For this review, take the finished solid that the model builds, in its own axes (mm). Coordinates: 2 decimals unless noted, no trailing zeros. Loops run counter-clockwise (first coordinate to the right, second up) from the corner with the lowest first, then second, coordinate; pieces in that order, holes last. Notation, with made-up numbers: (76.5, 5) - (105.5, 5) arc R32 ccw to (105.5, 33) - close; hole circle Ø2 at (56, -26.75). An arc over 180 degrees is marked (long way). One line per item, written item: value. Start each with the question number.
1. To check wall thickness, follow line 1 (Y direction, x = 0, z = 8.75) (3 decimals); line 2 (Y direction, x = 0, z = 10.25) (3 decimals); line 3 (Z direction, x = -1.5, y = -0.5). State the ranges of each line that lie inside material, in increasing order. Write a range as from..to.
2. Insertion check: pin 1 (7 mm diameter, centred on x = 0, y = 0, fed in from +Z); pin 2 (6 mm diameter, centred on x = 1, y = -2.5, fed in from +Z); pin 3 (3 mm diameter, centred on y = -4.5, z = 5.5, fed in from +X); pin 4 (6 mm diameter, centred on y = -2, z = 0, fed in from +X). Each pin has a flat end and moves straight along its axis. Give the tip position at first contact, or say it passes through.
3. Take a section at D-D, the plane z = -0.5. State the section outline as (x, y) points, and give its area (3 significant figures).
4. Take a section at C-C, the plane z = 4.75. State the section outline as (x, y) points (3 decimals).
5. Take a section at A-A, the plane y = 0. State the section outline as (x, z) points (3 decimals).
6. The part is to be moulded in two halves that separate along Y. For faces 1 (the face through (0, 0, 4)), 2 (the face through (4, -4, 9)), 3 (the face through (6.466, 2.681, 10.479)), 4 (the face through (4.125, 1.299, 8.056)), say which applies: released by +Y, released by -Y, zero draft, split by the parting line, or undercut.
Autodesk Inventor part; units mm, degrees
ref_plane "YZ Plane" through (0, 0, 0) normal (1, 0, 0) x (0, 1, 0)
ref_plane "XZ Plane" through (0, 0, 0) normal (0, 1, 0) x (-1, 0, 0)
ref_plane "XY Plane" through (0, 0, 0) normal (0, 0, 1) x (1, 0, 0)
sketch "Sketch5" plane through (0, 0, 0) normal (0, 0, 1) x (1, 0, 0)
  circle A0 centre (0, 0) radius 5.45
  dimension "d0" = 10.9
extrude "Extrusion1" add sketch "Sketch5" along normal blind 9
sketch "Sketch6" plane through (0, 0, 9) normal (0, 0, 1) x (1, 0, 0)
  circle A0 centre (0, 0) radius 7
  dimension "d3" = 14
extrude "Extrusion2" add sketch "Sketch6" along normal blind 3
sketch "Sketch7" plane through (0, 0, 12) normal (0, 0, 1) x (1, 0, 0)
  circle A0 centre (0, 0) radius 4.325
  dimension "d6" = 8.65
extrude "Extrusion3" cut sketch "Sketch7" against normal blind 8
sketch "Sketch8" plane through (0, 0, 0) normal (0, 0, -1) x (-1, 0, 0)
  circle A0 centre (0, 0) radius 5.45
  dimension "d9" = 10.9
extrude "Extrusion4" add sketch "Sketch8" along normal blind 5
properties part number "zaślepka"
Solutions:
1. line 1: -5.45..-4.325, 4.325..5.45
1. line 2: -7..-4.325, 4.325..7
1. line 3: -5..4
2. pin 1: z = 4
2. pin 2: z = 12
2. pin 3: x = 4.55
2. pin 4: x = 5.45
3. outline: circle Ø10.9 at (0, 0)
3. area: 93.3 mm2
4. outline: circle Ø10.9 at (0, 0); hole circle Ø8.65 at (0, 0)
5. outline: (-7, 9) - (-5.45, 9) - (-5.45, -5) - (5.45, -5) - (5.45, 9) - (7, 9) - (7, 12) - (4.325, 12) - (4.325, 4) - (-4.325, 4) - (-4.325, 12) - (-7, 12) - close
6. face 1: undercut
6. face 2: zero draft
6. face 3: split by the parting line
6. face 4: undercut
